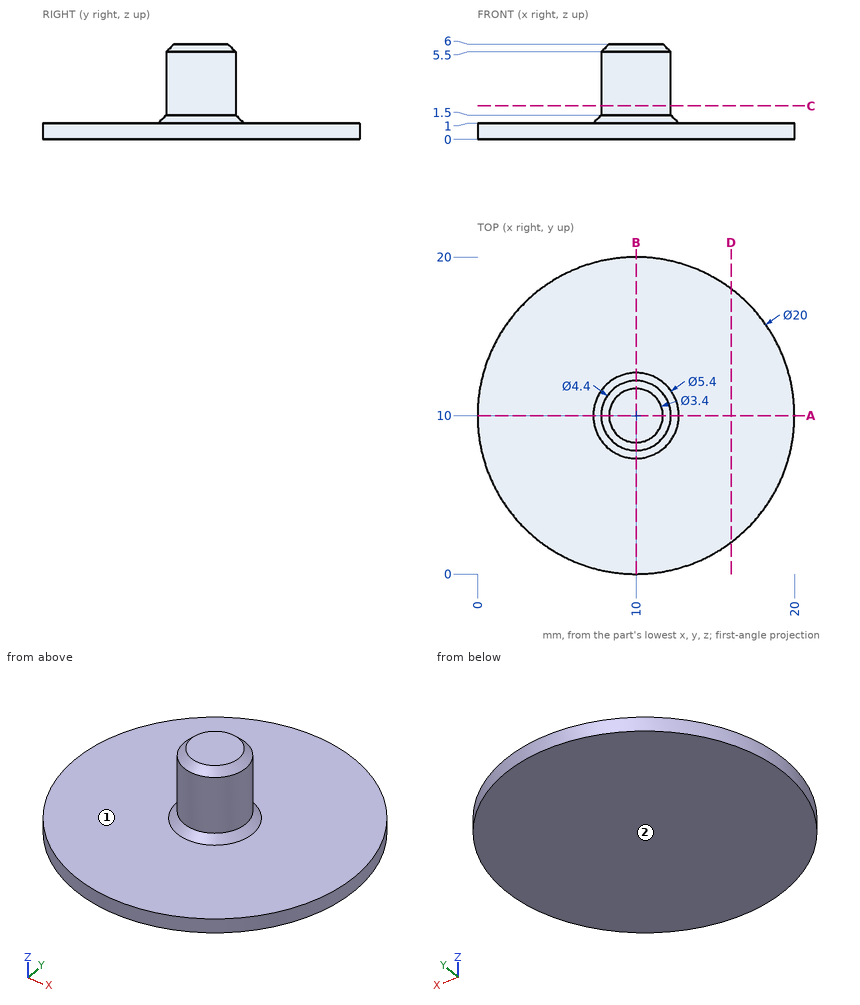
The figure shows three views and two pictorial views of one solid part (mm, origin at its lowest corner). Answer the questions. A direction names the side the tool comes from. Coordinates: 2 decimals unless noted, no trailing zeros. Write each loop counter-clockwise with the first axis right and the second up, starting at its lowest first coordinate (ties: lowest second). Pieces come first, ordered by that corner, then holes. Notation, with made-up numbers: (-35, 7) -> (14, 7) arc R10 cw to (14, 11) -> close; hole circle Ø1 at (35.5, 17). An arc over 180 degrees is marked (long way). Return JSON: item names as keys, results as strings.
(1) Consider line 1 along Z through (x, y) = (16.5, 16.75); line 2 along Y through (x, z) = (10.5, 4.85); line 3 along X through (y, z) = (7.5, 0.9). Determine where each line is inside the solid, lowest interval first. Write a range as from..to.
Answers below:
{"line 1": "0..1", "line 2": "7.86..12.14", "line 3": "0.32..19.68"}
(2) The part is cut by section A-A on y = 10. Give the vertices of the cut face in (x, z).
Answers below:
{"outline": "(0, 0) -> (20, 0) -> (20, 1) -> (12.7, 1) -> (12.2, 1.5) -> (12.2, 5.5) -> (11.7, 6) -> (8.3, 6) -> (7.8, 5.5) -> (7.8, 1.5) -> (7.3, 1) -> (0, 1) -> close"}
(3) The part is cut by section C-C on z = 2.1. Give the vertices of the cut face in (x, y), then the cut area to 3 significant figures.
Answers below:
{"outline": "circle Ø4.4 at (10, 10)", "area": "15.2 mm^2"}
(4) The part is cut by section D-D on x = 16. Give the vertices of the cut face in (y, z).
Answers below:
{"outline": "(2, 0) -> (18, 0) -> (18, 1) -> (2, 1) -> close"}
(5) Each of these flat-tipped pins is pushed along its axis until it touches: P1, Ø1.5, axis at x = 11.5, z = 4, coming from the -Y side; P2, Ø3, axis at x = 6, z = 0.5, coming from the +Y side; P3, Ø1.5, axis at y = 5.5, z = 1, coming from the +X side. Where does it stop, or does it pass through?
Answers below:
{"P1": "y = 7.93", "P2": "y = 19.68", "P3": "x = 19.27"}
(6) Which of the six approach directions +Z, -Z, +X, -X, +Y, -Y give full straight-line access (tool end or side, diameter ignored) to the marked faces 1 and 2?
Answers below:
{"face 1": "+Z", "face 2": "-Z, +X, -X, +Y, -Y"}
